from build123d import *

# Parameters (mm, degrees)
BOSS_EXTRUDE1_DEPTH = 2


with BuildPart() as part:
    # Sketch1 → Boss-Extrude1 (new body)
    with BuildSketch(Plane(origin=(0, 0, 0), x_dir=(1, 0, 0), z_dir=(0, 1, 0))):
        with BuildLine():
            Line((-29.21, 67.31), (29.21, 67.31))
            Line((29.21, 67.31), (29.21, 22.7))
            ThreePointArc((29.21, 22.7), (32.138932188, 15.628932188), (39.21, 12.7))
            Line((39.21, 12.7), (54.61, 12.7))
            Line((54.61, 12.7), (54.61, -12.7))
            Line((54.61, -12.7), (39.21, -12.7))
            ThreePointArc((39.21, -12.7), (32.138932188, -15.628932188), (29.21, -22.7))
            Line((29.21, -22.7), (29.21, -67.31))
            Line((29.21, -67.31), (-29.21, -67.31))
            Line((-29.21, -67.31), (-29.21, 67.31))
        make_face()
    extrude(amount=BOSS_EXTRUDE1_DEPTH)


solid = part.part
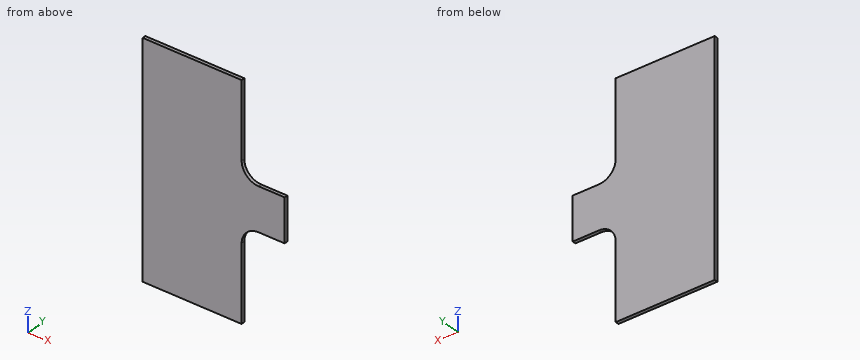
Geometry check sheet. Reference: the model listing, model coordinates, mm. Round coordinates to 2 decimals unless told otherwise and drop trailing zeros. Loops run counter-clockwise (first coordinate to the right, second up) from the corner with the lowest first, then second, coordinate; pieces in that order, holes last. Notation, with made-up numbers: (54.5, 44.25) -> (75.5, 44.25) arc R20 cw to (75.5, 76.25) -> close; hole circle Ø8 at (47, 19). An arc over 180 degrees is marked (long way). Answer as a JSON object with one key per item and string values. Group by question number.
Item 1: Thickness scan on line 1 along Z through (x, y) = (41, 0.2); line 2 along X through (y, z) = (0.45, 37); line 3 along X through (y, z) = (1.5, -15). Record the ranges inside material, lowest first.
Item 2: Cross-section at C-C, the plane z = -46. Record the cut outline in (x, y), plus the area to 3 significant figures.
Item 3: Depth check by flat-ended pin: pin 1 Ø0.6 at (x, y) = (50.5, 0.5) entering from -Z; pin 2 Ø0.6 at (y, z) = (1.5, 44.5) entering from +X. Enter the tip coordinate at first touch or a pass-through.
Item 4: Cross-section at A-A, the plane y = 1.2. Record the cut outline in (x, z).
Item 5: Cross-section at B-B, the plane x = 42. Record the cut outline in (y, z), plus the area to 3 significant figures.
Determined:
{
 "1": {"line 1": "z = -12.7 to 12.7", "line 2": "x = -29.21 to 29.21", "line 3": "x = -29.21 to 32.83"},
 "2": {"outline": "(-29.21, 0) -> (29.21, 0) -> (29.21, 2) -> (-29.21, 2) -> close", "area": "117 mm²"},
 "3": {"pin 1": "stops at z = -12.7", "pin 2": "stops at x = 29.21"},
 "4": {"outline": "(-29.21, -67.31) -> (29.21, -67.31) -> (29.21, -22.7) arc R10 cw to (39.21, -12.7) -> (54.61, -12.7) -> (54.61, 12.7) -> (39.21, 12.7) arc R10 cw to (29.21, 22.7) -> (29.21, 67.31) -> (-29.21, 67.31) -> close"},
 "5": {"outline": "(0, -12.7) -> (2, -12.7) -> (2, 12.7) -> (0, 12.7) -> close", "area": "50.8 mm²"}
}
